Can you work these out from the model? Positions are in its coordinate system, mm. A direction names the side the tool comes from. Give positions to 0.01 mm unless a question says otherwise; leave off trailing zeros. Order: outer loops, then holes, each group sorted by start corner. A loop starts at its lowest first (then second) coordinate and runs counter-clockwise, first axis right, second up. Notation, with made-up numbers: M 65.25,-22 L 77.25,-22 A17 ccw 77.25,0 Z; hole C 60,83.5 d6. An arc over 180 degrees is marked long. Write each question's results on one line, items separated by ' | '.
from build123d import *

# Parameters (mm, degrees)
SKETCH_1_R               = 7.5
EXTRUDE_1_DEPTH          = 3.5
SKETCH_2_R               = 6.115
EXTRUDE_2_DEPTH          = 7
CUT_EXTRUDE_3_DEPTH      = 7
SKETCH_3_R               = 7.5
EXTRUDE_3_DEPTH          = 1
SKETCH_6_R               = 2
CUT_EXTRUDE_2_DEPTH      = 16
PATTERN_CIRCULAR_2_COUNT = 20
SKETCH_13_W              = 1.25
SKETCH_13_H              = 7.5
PATTERN_CIRCULAR_4_COUNT = 2
PATTERN_CIRCULAR_4_ANGLE = 90


with BuildPart() as part:
    # 草圖1 → 填料-伸長1 (new body, symmetric)
    with BuildSketch(Plane.XY):
        Circle(SKETCH_1_R)
    extrude(amount=EXTRUDE_1_DEPTH, both=True)

    # 草圖2 → 填料-伸長2 (add)
    with BuildSketch(Plane.XY.offset(3.5)):
        Circle(SKETCH_2_R)
    extrude(amount=EXTRUDE_2_DEPTH)

    # 草圖7 → 除料-伸長3 (cut)
    with BuildSketch(Plane.XY.offset(10.5)):
        with BuildLine():
            ThreePointArc((-0.599277509, 6.085564186), (0, 5.515), (0.599277509, 6.085564186))
            ThreePointArc((0.599277509, 6.085564186), (0, 6.115), (-0.599277509, 6.085564186))
        make_face()
    cut_extrude_3 = extrude(amount=-CUT_EXTRUDE_3_DEPTH, mode=Mode.SUBTRACT)

    # 草圖3 → 填料-伸長3 (add)
    with BuildSketch(Plane.XY.offset(10.5)):
        Circle(SKETCH_3_R)
    extrude(amount=EXTRUDE_3_DEPTH)

    # 草圖6 → 除料-伸長2 (cut, through all)
    with BuildSketch(Plane(origin=(0, 0, -3.5), x_dir=(-1, 0, 0), z_dir=(0, 0, -1))):
        Circle(SKETCH_6_R)
    extrude(amount=-CUT_EXTRUDE_2_DEPTH, mode=Mode.SUBTRACT)

    # 環狀複製排列2: 除料-伸長3 ×20 about axis
    pattern_circular_2_axis = Axis((0, 0, 0), (0, 0, 1))
    for i in range(1, PATTERN_CIRCULAR_2_COUNT):
        add(cut_extrude_3.rotate(pattern_circular_2_axis, i * 360 / PATTERN_CIRCULAR_2_COUNT), mode=Mode.SUBTRACT)

    # 草圖13 → M3x0.5 螺紋孔3 (revolve, cut)
    with BuildSketch(Plane(origin=(0, 0, 0), x_dir=(0, 0, -1), z_dir=(1, 0, 0))):
        with Locations((0.625, 3.75)):
            Rectangle(SKETCH_13_W, SKETCH_13_H)
    m3x0_5_3 = revolve(axis=Axis((0, -6.35, 0), (0, 1, 0)), mode=Mode.SUBTRACT)

    # 環狀複製排列4: M3x0.5 螺紋孔3 ×2 about axis
    pattern_circular_4_axis = Axis((0, 0, 3.5), (0, 0, 1))
    for i in range(1, PATTERN_CIRCULAR_4_COUNT):
        add(m3x0_5_3.rotate(pattern_circular_4_axis, i * PATTERN_CIRCULAR_4_ANGLE / (PATTERN_CIRCULAR_4_COUNT - 1)), mode=Mode.SUBTRACT)


solid = part.part
(1) Will these pins go through, and if not, where does the flat tip stop? P1, Ø6, axis at x = 5, z = 3.5, coming from the -Y side; P2, Ø1.5, axis at x = 3, z = 10, coming from the -Y side; P3, Ø1.5, axis at y = 0, z = 0, coming from the -X side.
Data:
P1: stops at y = -7.23 | P2: stops at y = -7.09 | P3: stops at x = 1.85
(2) We'd pull the mould along Z, two halves only. Please class faces 4 (the face through (2, -2, 11.5)), 5 (the face through (-0.013, 5.515, 7.049)): +Z half, -Z half, draft (parallel to the pull), parting line (faces both ways), or undercut.
Data:
face 4: +Z half | face 5: undercut
(3) I need wall thicknesses on L1, parallel to Z at x = 0, y = 5.6; L2, parallel to Y at x = 0, z = 8 (3 decimals); L3, parallel to Z at x = 7.25, y = -0.5. Which ranges of each line are inside material? Lowest first, please. Write a range as from..to.
Data:
L1: z = -3.5..-1.25, 1.25..3.5, 10.5..11.5 | L2: y = -5.515..-2, 2..5.515 | L3: z = -3.5..3.5, 10.5..11.5
(4) For faces 1 (the face through (-4.57, -0.05, 1.25)), 2 (the face through (5.515, 0.013, 7.049)), 3 (the face through (3.23, 4.47, 7.05)), which set-ups out of +Z, -Z, +X, -X, +Y, -Y let a thin tool reach every point of the face, with its end or its side?
Data:
face 1: -X | face 2: +X | face 3: none
(5) Imagine slicing it at A-A, the plane x = 0. Write out the boundary of the cut face in (y, z) (3 decimals).
Data:
outline: M -7.5,-3.5 L -2,-3.5 L -2,11.5 L -7.5,11.5 L -7.5,10.5 L -5.515,10.5 L -5.515,3.5 L -7.5,3.5 Z; M 2,-3.5 L 7.5,-3.5 L 7.5,-1.25 L 2,-1.25 Z; M 2,1.25 L 7.5,1.25 L 7.5,3.5 L 5.515,3.5 L 5.515,10.5 L 7.5,10.5 L 7.5,11.5 L 2,11.5 Z
(6) Imagine slicing it at D-D, the plane y = 2.75. Write out the boundary of the cut face in (x, z), plus the area to 3 significant figures.
Data:
outline: M -6.98,-3.5 L 6.98,-3.5 L 6.98,3.5 L 5.46,3.5 L 5.46,10.5 L 6.98,10.5 L 6.98,11.5 L -6.98,11.5 L -6.98,10.5 L -5.46,10.5 L -5.46,3.5 L -6.98,3.5 Z; hole C 0,0 d2.5 | area: 183 mm2
(7) Imagine slicing it at C-C, the plane z = 0. Write out the boundary of the cut face in (x, y).
Data:
outline: M -7.4,-1.25 A7.5 ccw long 1.25,7.4 L 1.25,1.56 A2 cw long -1.56,-1.25 Z; M -7.4,1.25 L -1.56,1.25 A2 cw -1.25,1.56 L -1.25,7.4 A7.5 ccw Z
(8) Imagine slicing it at B-B, the plane y = 0. Write out the boundary of the cut face in (x, z) (3 decimals), plus the area to 3 significant figures.
Data:
outline: M -7.5,-3.5 L -2,-3.5 L -2,-1.25 L -7.5,-1.25 Z; M -7.5,1.25 L -2,1.25 L -2,11.5 L -7.5,11.5 L -7.5,10.5 L -5.515,10.5 L -5.515,3.5 L -7.5,3.5 Z; M 2,-3.5 L 7.5,-3.5 L 7.5,3.5 L 5.515,3.5 L 5.515,10.5 L 7.5,10.5 L 7.5,11.5 L 2,11.5 Z | area: 123 mm2
